Input: part model. Units: mm. Frame: model coordinates. Coordinates: 2 decimals unless noted, no trailing zeros. Order: outer loops, then holes, each group sorted by start corner. A loop starts at its lowest first (then second) coordinate and runs counter-clockwise, first axis right, second up. Notation, with made-up numbers: (-15.5, 63.5) -> (2.5, 63.5) arc R19 ccw to (2.5, 83.5) -> close; hole circle Ø6 at (44, 1). An arc over 180 degrees is marked (long way). Answer as CSV lines item,"result".
from build123d import *

# Parameters (mm, degrees)
CROQUIS2_R              = 65
SALIENTE_EXTRUIR1_DEPTH = 4
CORTAR_EXTRUIR6_REACH   = 94.011
CROQUIS3_W              = 4
CROQUIS3_H              = 10.2
CROQUIS4_W              = 23
CROQUIS4_H              = 42
CORTAR_EXTRUIR8_DEPTH   = 10


with BuildPart() as part:
    # Croquis2 → Saliente-Extruir1 (new body)
    with BuildSketch(Plane(origin=(0, 0, 0), x_dir=(1, 0, 0), z_dir=(0, 1, 0))):
        with Locations(Location((0, 0, 0), (0, 0, 270))):
            Circle(CROQUIS2_R)
    extrude(amount=SALIENTE_EXTRUIR1_DEPTH)

    # Croquis3 → Cortar-Extruir6 (cut, up to next)
    with BuildSketch(Plane(origin=(0, 4, 0), x_dir=(1, 0, 0), z_dir=(0, 1, 0)), mode=Mode.PRIVATE) as cortar_extruir6_sk1:
        with Locations((-37, 12.5)):
            Rectangle(CROQUIS3_W, CROQUIS3_H)
    cortar_extruir6_tool1 = extrude(cortar_extruir6_sk1.sketch, amount=-CORTAR_EXTRUIR6_REACH, mode=Mode.PRIVATE) & part.part
    # Croquis3 → Cortar-Extruir6 (cut, up to next)
    with BuildSketch(Plane(origin=(0, 4, 0), x_dir=(1, 0, 0), z_dir=(0, 1, 0)), mode=Mode.PRIVATE) as cortar_extruir6_sk2:
        with Locations((-37, -12.7)):
            Rectangle(CROQUIS3_W, CROQUIS3_H)
    cortar_extruir6_tool2 = extrude(cortar_extruir6_sk2.sketch, amount=-CORTAR_EXTRUIR6_REACH, mode=Mode.PRIVATE) & part.part
    # Croquis3 → Cortar-Extruir6 (cut, up to next)
    with BuildSketch(Plane(origin=(0, 4, 0), x_dir=(1, 0, 0), z_dir=(0, 1, 0)), mode=Mode.PRIVATE) as cortar_extruir6_sk3:
        with Locations((-37, -37.9)):
            Rectangle(CROQUIS3_W, CROQUIS3_H)
    cortar_extruir6_tool3 = extrude(cortar_extruir6_sk3.sketch, amount=-CORTAR_EXTRUIR6_REACH, mode=Mode.PRIVATE) & part.part
    # Croquis3 → Cortar-Extruir6 (cut, up to next)
    with BuildSketch(Plane(origin=(0, 4, 0), x_dir=(1, 0, 0), z_dir=(0, 1, 0)), mode=Mode.PRIVATE) as cortar_extruir6_sk4:
        with Locations((-37, 37.7)):
            Rectangle(CROQUIS3_W, CROQUIS3_H)
    cortar_extruir6_tool4 = extrude(cortar_extruir6_sk4.sketch, amount=-CORTAR_EXTRUIR6_REACH, mode=Mode.PRIVATE) & part.part
    # Croquis3 → Cortar-Extruir6 (cut, up to next)
    with BuildSketch(Plane(origin=(0, 4, 0), x_dir=(1, 0, 0), z_dir=(0, 1, 0)), mode=Mode.PRIVATE) as cortar_extruir6_sk5:
        with Locations((37, 37.7)):
            Rectangle(CROQUIS3_W, CROQUIS3_H)
    cortar_extruir6_tool5 = extrude(cortar_extruir6_sk5.sketch, amount=-CORTAR_EXTRUIR6_REACH, mode=Mode.PRIVATE) & part.part
    # Croquis3 → Cortar-Extruir6 (cut, up to next)
    with BuildSketch(Plane(origin=(0, 4, 0), x_dir=(1, 0, 0), z_dir=(0, 1, 0)), mode=Mode.PRIVATE) as cortar_extruir6_sk6:
        with Locations((37, 12.5)):
            Rectangle(CROQUIS3_W, CROQUIS3_H)
    cortar_extruir6_tool6 = extrude(cortar_extruir6_sk6.sketch, amount=-CORTAR_EXTRUIR6_REACH, mode=Mode.PRIVATE) & part.part
    # Croquis3 → Cortar-Extruir6 (cut, up to next)
    with BuildSketch(Plane(origin=(0, 4, 0), x_dir=(1, 0, 0), z_dir=(0, 1, 0)), mode=Mode.PRIVATE) as cortar_extruir6_sk7:
        with Locations((37, -12.7)):
            Rectangle(CROQUIS3_W, CROQUIS3_H)
    cortar_extruir6_tool7 = extrude(cortar_extruir6_sk7.sketch, amount=-CORTAR_EXTRUIR6_REACH, mode=Mode.PRIVATE) & part.part
    # Croquis3 → Cortar-Extruir6 (cut, up to next)
    with BuildSketch(Plane(origin=(0, 4, 0), x_dir=(1, 0, 0), z_dir=(0, 1, 0)), mode=Mode.PRIVATE) as cortar_extruir6_sk8:
        with Locations((37, -37.9)):
            Rectangle(CROQUIS3_W, CROQUIS3_H)
    cortar_extruir6_tool8 = extrude(cortar_extruir6_sk8.sketch, amount=-CORTAR_EXTRUIR6_REACH, mode=Mode.PRIVATE) & part.part
    add(cortar_extruir6_tool1.solids().sort_by_distance((-37, 4, -12.5))[0], mode=Mode.SUBTRACT)
    add(cortar_extruir6_tool2.solids().sort_by_distance((-37, 4, 12.7))[0], mode=Mode.SUBTRACT)
    add(cortar_extruir6_tool3.solids().sort_by_distance((-37, 4, 37.9))[0], mode=Mode.SUBTRACT)
    add(cortar_extruir6_tool4.solids().sort_by_distance((-37, 4, -37.7))[0], mode=Mode.SUBTRACT)
    add(cortar_extruir6_tool5.solids().sort_by_distance((37, 4, -37.7))[0], mode=Mode.SUBTRACT)
    add(cortar_extruir6_tool6.solids().sort_by_distance((37, 4, -12.5))[0], mode=Mode.SUBTRACT)
    add(cortar_extruir6_tool7.solids().sort_by_distance((37, 4, 12.7))[0], mode=Mode.SUBTRACT)
    add(cortar_extruir6_tool8.solids().sort_by_distance((37, 4, 37.9))[0], mode=Mode.SUBTRACT)

    # Croquis4 → Cortar-Extruir8 (cut)
    with BuildSketch(Plane(origin=(0, 4, 0), x_dir=(1, 0, 0), z_dir=(0, 1, 0))):
        with Locations((0, 10)):
            Rectangle(CROQUIS4_W, CROQUIS4_H)
    extrude(amount=-CORTAR_EXTRUIR8_DEPTH, mode=Mode.SUBTRACT)


solid = part.part
1. Cut plane A-A (z = 0). Return the cut outline in (x, y), plus the area to 3 significant figures.
Findings:
outline,"(-65, 0) -> (-11.5, 0) -> (-11.5, 4) -> (-65, 4) -> close; (11.5, 0) -> (65, 0) -> (65, 4) -> (11.5, 4) -> close"
area,"428 mm2"
2. Cut plane C-C (y = 0.75). State how many separate pieces and enclosed holes the cut face has, plus the area to 3 significant figures.
Findings:
separate pieces,"1"
enclosed holes,"9"
area,"12,000 mm2"
3. Cut plane B-B (x = 0). Return the cut outline in (y, z), plus the area to 3 significant figures.
Findings:
outline,"(0, -65) -> (4, -65) -> (4, -31) -> (0, -31) -> close; (0, 11) -> (4, 11) -> (4, 65) -> (0, 65) -> close"
area,"352 mm2"
4. Mould query, pull axis Z, two halves, no side actions, for faces 1 (the face through (19.52, 1.97, 62)), 2 (the face through (35, 2, 38)). Classes: released by +Z, released by -Z, zero draft, split by the parting line, or undercut.
Findings:
face 1,"split by the parting line"
face 2,"undercut"
5. Ray query, line 1 along X through (y, z) = (2.3, 1.5); line 2 along X through (y, z) = (2, 13); line 3 along X through (y, z) = (1.45, -36). Return the intervals inside material, ascending.
Findings:
line 1,"x = -64.98 to -11.5, 11.5 to 64.98"
line 2,"x = -63.69 to -39, -35 to 35, 39 to 63.69"
line 3,"x = -54.12 to -39, -35 to 35, 39 to 54.12"
6. Cut plane D-D (x = -53.5). Return the cut outline in (y, z).
Findings:
outline,"(0, -36.92) -> (4, -36.92) -> (4, 36.92) -> (0, 36.92) -> close"
7. Contact query for flat-ended pins moving along their axis: pin 1 (1 mm diameter, centred on y = 2, z = -36.5, fed in from -X); pin 2 (2 mm diameter, centred on x = -37.5, y = 2, fed in from -Z); pin 3 (1.2 mm diameter, centred on y = 1.5, z = -7.5, fed in from +X). Output: stop coordinate, or through.
Findings:
pin 1,"stops at x = -54.12"
pin 2,"stops at z = -53.78"
pin 3,"stops at x = 64.63"
